Verification items for the finished model (mm, model axes). Face numbers are marked on the shaded views. A direction names the side the tool comes from. Coordinates: 2 decimals unless noted, no trailing zeros. Order: outer loops, then holes, each group sorted by start corner. A loop starts at its lowest first (then second) coordinate and runs counter-clockwise, first axis right, second up.
Q1. Depth check by flat-ended pin: P1, Ø5, axis at x = 29, y = 10, coming from the +Z side; P2, Ø1.5, axis at x = 32, z = -9.5, coming from the -Y side; P3, Ø5, axis at x = -26, z = -25, coming from the +Y side; P4, Ø5, axis at x = -31.925, z = 9, coming from the -Y side. Enter the tip coordinate at first touch or a pass-through.
Q2. Cross-section at C-C, the plane y = 8.5. Record the boundary of the cut face in (x, z), and give its area (3 significant figures).
Q3. Cross-section at D-D, the plane x = -37.5. Record the boundary of the cut face in (y, z), and give its area (3 significant figures).
Q4. Set-up check for the marked faces 1 and 2: record each of +Z, -Z, +X, -X, +Y, -Y from which the full face is reachable in a straight line by a thin tool's end or side.
Q5. Cross-section at B-B, the plane x = 0. Record the boundary of the cut face in (y, z), and give its area (3 significant figures).
Q6. Thickness scan on line 1 (X direction, y = 4.25, z = 9) (3 decimals); line 2 (X direction, y = 5.5, z = -1.5); line 3 (Y direction, x = -34, z = 13.5). Record the ranges inside material, lowest first.
Q7. Cross-section at A-A, the plane z = 0. Record the boundary of the cut face in (x, y).
from build123d import *

# Parameters (mm, degrees)
SKETCH_2_R          = 50
EXTRUDE_1_DEPTH     = 15
SKETCH_5_R          = 20
EXTRUDE_2_DEPTH     = 10
SKETCH_6_R          = 1.5
CUT_EXTRUDE_1_DEPTH = 7


with BuildPart() as part:
    # Эскиз2 → Бобышка-Вытянуть1 (new body)
    with BuildSketch(Plane(origin=(0, 0, 0), x_dir=(1, 0, 0), z_dir=(0, 1, 0))):
        with Locations(Location((0, 0, 0), (0, 0, 270))):
            Circle(SKETCH_2_R)
    extrude(amount=EXTRUDE_1_DEPTH)

    # Эскиз5 → Бобышка-Вытянуть2 (add)
    with BuildSketch(Plane(origin=(0, 15, 0), x_dir=(1, 0, 0), z_dir=(0, 1, 0))):
        with Locations(Location((0, 0, 0), (0, 0, 270))):
            Circle(SKETCH_5_R)
    extrude(amount=EXTRUDE_2_DEPTH)

    # Эскиз6 → Вырез-Вытянуть1 (cut)
    with BuildSketch(Plane.XZ):
        with Locations(Location((31.93, 9, 0), (0, 0, 270))):
            Circle(SKETCH_6_R)
        with Locations(Location((31.93, -9, 0), (0, 0, 270))):
            Circle(SKETCH_6_R)
        with Locations(Location((-31.925, 9, 0), (0, 0, 270))):
            Circle(SKETCH_6_R)
        with Locations(Location((-31.925, -9, 0), (0, 0, 270))):
            Circle(SKETCH_6_R)
    extrude(amount=-CUT_EXTRUDE_1_DEPTH, mode=Mode.SUBTRACT)


solid = part.part
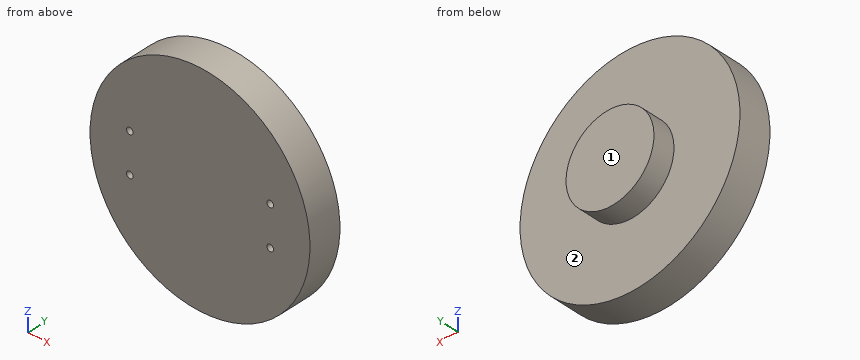
Check values:
1. P1: stops at z = 42.4
1. P2: stops at y = 7
1. P3: stops at y = 15
1. P4: stops at y = 0
2. outline: circle Ø100 at (0, 0)
2. area: 7,850 mm2
3. outline: (0, -33.07) - (15, -33.07) - (15, 33.07) - (0, 33.07) - close
3. area: 992 mm2
4. face 1: +Z, -Z, +X, -X, +Y
4. face 2: +Y
5. outline: (0, -50) - (15, -50) - (15, -20) - (25, -20) - (25, 20) - (15, 20) - (15, 50) - (0, 50) - close
5. area: 1,900 mm2
6. line 1: x = -49.183 to -33.425, -30.425 to 30.43, 33.43 to 49.183
6. line 2: x = -49.98 to 49.98
6. line 3: y = 0 to 15
7. outline: (-50, 0) - (50, 0) - (50, 15) - (20, 15) - (20, 25) - (-20, 25) - (-20, 15) - (-50, 15) - close
